Input: dimensioned drawing with shaded views. Units: mm. Origin: part minimum x, y, z. A direction names the side the tool comes from. Coordinates: 2 decimals unless noted, no trailing zeros. Order: outer loops, then holes, each group sorted by start corner. A loop starts at its lowest first (then second) coordinate and runs counter-clockwise, first axis right, second up. Notation, with made-up numbers: (49, 71) -> (80, 71) arc R17 ccw to (80, 102) -> close; hole circle Ø1 at (5, 48.25). An arc over 180 degrees is marked (long way). Answer in a Markdown table with one row per item. Add a question column.
1) Pull-direction query (Z, two-part tool) for the marked faces 1 and 2; classes: +Z half, -Z half, draft (parallel to the pull), parting line (faces both ways), or undercut.
2) Section query B-B on z = 6. Return the cut outline in (x, y).
3) Section query D-D on x = 1. Return the cut outline in (y, z), then the cut area to 3 significant figures.
4) Contact query for flat-ended pins moving along their axis: P1, Ø5, axis at x = 8.5, y = 9, coming from the -Z side; P2, Ø2, axis at x = 2.5, y = 6, coming from the +Z side; P3, Ø2, axis at x = 9, y = 4, coming from the -Z side. Output: stop coordinate, or through.
5) Set-up query: the marked faces 3 and 4. Return all of +Z, -Z, +X, -X, +Y, -Y with unobstructed straight access to the full face (end or side cutting, diameter ignored); none if empty.
6) Section query A-A on x = 6. Return the cut outline in (y, z), then the cut area to 3 significant figures.
7) Section query C-C on y = 6.5. Return the cut outline in (x, z), then the cut area to 3 significant figures.
8) Ray query, line 1 (Y direction, x = 3.5, z = 10); line 2 (Z direction, x = 7.75, y = 4); line 3 (Z direction, x = 4, y = 2.75). Return the intervals inside material, ascending. Write a range as from..to.
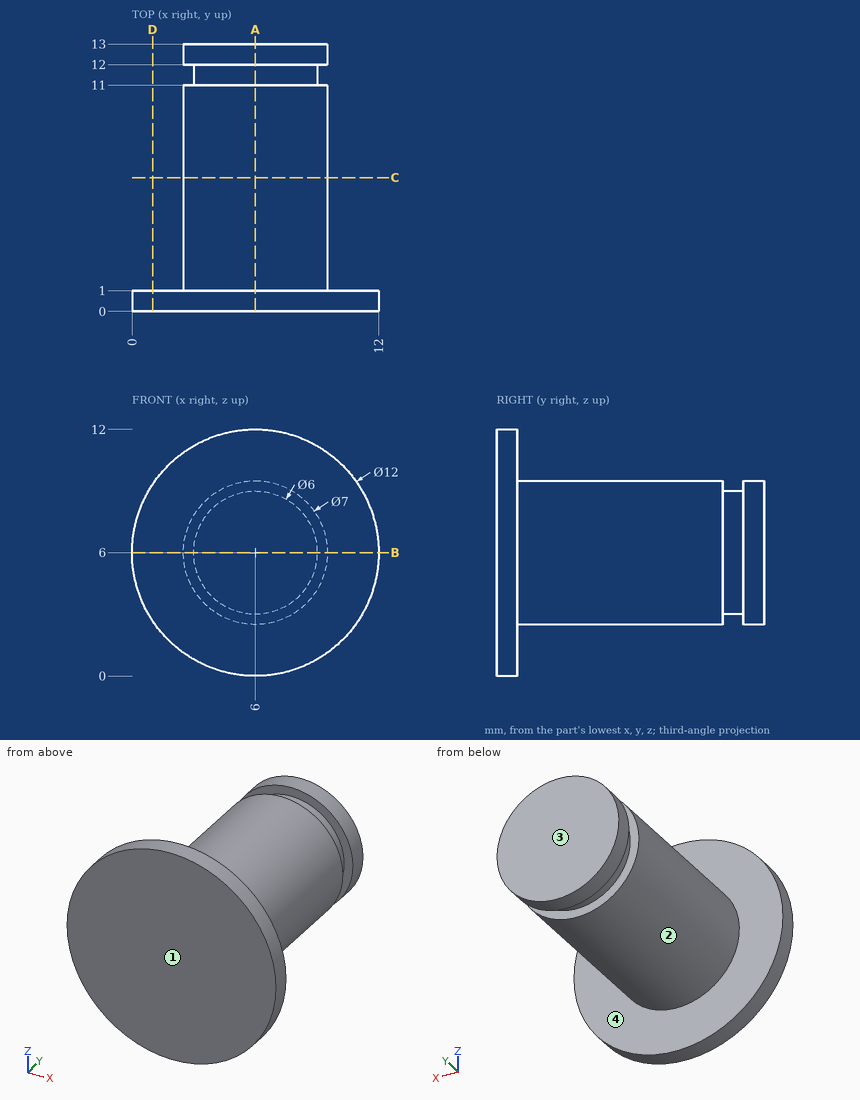
Result:
| question | item | result |
|---|---|---|
| 1 | face 1 | draft |
| 1 | face 2 | parting line |
| 2 | outline | (0, 0) -> (12, 0) -> (12, 1) -> (9.5, 1) -> (9.5, 11) -> (9, 11) -> (9, 12) -> (9.5, 12) -> (9.5, 13) -> (2.5, 13) -> (2.5, 12) -> (3, 12) -> (3, 11) -> (2.5, 11) -> (2.5, 1) -> (0, 1) -> close |
| 3 | outline | (0, 2.68) -> (1, 2.68) -> (1, 9.32) -> (0, 9.32) -> close |
| 3 | area | 6.63 mm2 |
| 4 | P1 | z = 2.5 |
| 4 | P2 | z = 8.45 |
| 4 | P3 | z = 3.13 |
| 5 | face 3 | +Z, -Z, +X, -X, +Y |
| 5 | face 4 | +Y |
| 6 | outline | (0, 0) -> (1, 0) -> (1, 2.5) -> (11, 2.5) -> (11, 3) -> (12, 3) -> (12, 2.5) -> (13, 2.5) -> (13, 9.5) -> (12, 9.5) -> (12, 9) -> (11, 9) -> (11, 9.5) -> (1, 9.5) -> (1, 12) -> (0, 12) -> close |
| 6 | area | 95.0 mm2 |
| 7 | outline | circle Ø7 at (6, 6) |
| 7 | area | 38.5 mm2 |
| 8 | line 1 | 0..1 |
| 8 | line 2 | 2.97..9.03 |
| 8 | line 3 | 3.13..8.87 |
